from build123d import *

# Parameters (mm, degrees)
SKETCH1_W           = 164.845307866
SKETCH1_H           = 115.711925012
SKETCH1_W_2         = 150.387290324
SKETCH1_H_2         = 105.563228254
BOSS_EXTRUDE1_DEPTH = 2.54
SKETCH1_3_W         = 164.845307866
SKETCH1_3_H         = 115.711925012
SKETCH1_3_W_2       = 150.387290324
SKETCH1_3_H_2       = 105.563228254
BOSS_EXTRUDE2_DEPTH = 53.34
BOSS_EXTRUDE3_START = 53.34
SKETCH1_4_W         = 164.845307866
SKETCH1_4_H         = 115.711925012
SKETCH1_4_W_2       = 150.387290324
SKETCH1_4_H_2       = 105.563228254
BOSS_EXTRUDE3_DEPTH = 2.54
SKETCH2_R           = 31.968042231
SKETCH2_R_2         = 7.197604608
SKETCH2_R_3         = 7.702224934
SKETCH2_W           = 12.372659968
SKETCH2_H           = 29.724433098
CUT_EXTRUDE1_DEPTH  = 2.54
SKETCH3_W           = 4.472305678
SKETCH3_H           = 33.780947159
SKETCH3_W_2         = 4.478852124
SKETCH3_W_3         = 5.014326271
SKETCH3_W_4         = 5.285336568
SKETCH3_W_5         = 5.288609791
SKETCH3_W_6         = 4.762955313
SKETCH3_W_7         = 4.703323858
SKETCH3_W_8         = 4.457199363
CUT_EXTRUDE2_DEPTH  = 81.820687539


with BuildPart() as part:
    # Sketch1 → Boss-Extrude1 (new body)
    with BuildSketch(Plane(origin=(0, 0, 0), x_dir=(1, 0, 0), z_dir=(0, 1, 0))):
        Rectangle(SKETCH1_W, SKETCH1_H)
        Rectangle(SKETCH1_W_2, SKETCH1_H_2, mode=Mode.SUBTRACT)
        Rectangle(SKETCH1_W_2, SKETCH1_H_2)
    extrude(amount=BOSS_EXTRUDE1_DEPTH)

    # Sketch1<3> → Boss-Extrude2 (add)
    with BuildSketch(Plane(origin=(0, 0, 0), x_dir=(1, 0, 0), z_dir=(0, 1, 0))):
        Rectangle(SKETCH1_3_W, SKETCH1_3_H)
        Rectangle(SKETCH1_3_W_2, SKETCH1_3_H_2, mode=Mode.SUBTRACT)
    extrude(amount=BOSS_EXTRUDE2_DEPTH)

    # Sketch1<4> → Boss-Extrude3 (add)
    with BuildSketch(Plane(origin=(0, 0, 0), x_dir=(1, 0, 0), z_dir=(0, 1, 0)).offset(BOSS_EXTRUDE3_START)):
        Rectangle(SKETCH1_4_W, SKETCH1_4_H)
        Rectangle(SKETCH1_4_W_2, SKETCH1_4_H_2, mode=Mode.SUBTRACT)
        Rectangle(SKETCH1_4_W_2, SKETCH1_4_H_2)
    extrude(amount=BOSS_EXTRUDE3_DEPTH)

    # Sketch2 → Cut-Extrude1 (cut)
    with BuildSketch(Plane(origin=(0, 55.88, 0), x_dir=(1, 0, 0), z_dir=(0, 1, 0))):
        with Locations(Location((27.35736774, 0, 0), (0, 0, 270))):
            Circle(SKETCH2_R)
        with Locations(Location((-29.22455859, 32.289622442, 0), (0, 0, 270))):
            Circle(SKETCH2_R_2)
        with Locations(Location((-29.22455859, 3.70269924, 0), (0, 0, 270))):
            Circle(SKETCH2_R_2)
        with Locations(Location((-55.407149161, -25.489564673, 0), (0, 0, 270))):
            Circle(SKETCH2_R_3)
        with Locations((-55.407149161, 14.862216549)):
            Rectangle(SKETCH2_W, SKETCH2_H)
    extrude(amount=-CUT_EXTRUDE1_DEPTH, mode=Mode.SUBTRACT)

    # Sketch3 → Cut-Extrude2 (cut, along a direction that is not the sketch's normal)
    with BuildSketch(Plane.XY.offset(57.855962506)):
        with Locations((65.530463392, 25.643218911)):
            Rectangle(SKETCH3_W, SKETCH3_H)
        with Locations((56.86140712, 25.643218911)):
            Rectangle(SKETCH3_W_2, SKETCH3_H)
        with Locations((47.101763215, 25.643218911)):
            Rectangle(SKETCH3_W_3, SKETCH3_H)
        with Locations((37.06783579, 25.643218911)):
            Rectangle(SKETCH3_W_2, SKETCH3_H)
        with Locations((26.637212589, 25.643218911)):
            Rectangle(SKETCH3_W_4, SKETCH3_H)
        with Locations((16.066174405, 25.643218911)):
            Rectangle(SKETCH3_W_5, SKETCH3_H)
        with Locations((5.491862999, 25.643218911)):
            Rectangle(SKETCH3_W_6, SKETCH3_H)
        with Locations((-4.645950069, 25.643218911)):
            Rectangle(SKETCH3_W_7, SKETCH3_H)
        with Locations((-14.58703369, 25.643218911)):
            Rectangle(SKETCH3_W_8, SKETCH3_H)
    extrude(amount=-CUT_EXTRUDE2_DEPTH, dir=(0.7071067811865475, 0, 0.7071067811865477), mode=Mode.SUBTRACT)


solid = part.part
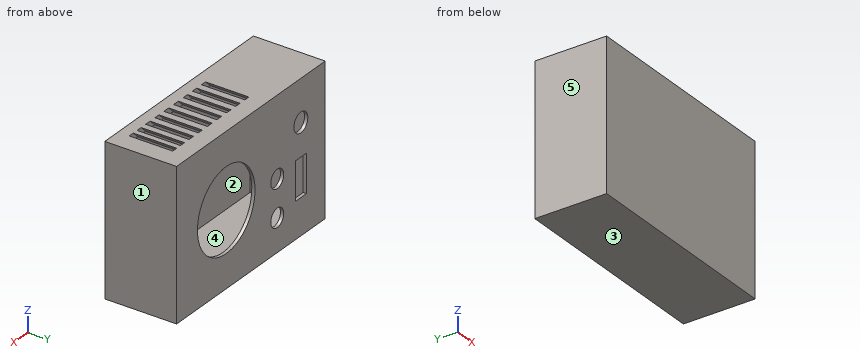
The listing builds one solid part. Answer for the finished solid, in the listing's coordinates (mm). Face numbers are marked on the shaded views. A direction names the side the tool comes from. Coordinates: 2 decimals unless noted, no trailing zeros. Order: outer loops, then holes, each group sorted by start corner. A loop starts at its lowest first (then second) coordinate and runs counter-clockwise, first axis right, second up. Notation, with made-up numbers: (81, 89.25) -> (106, 89.25) arc R35 ccw to (106, 125.25) -> close; hole circle Ø2 at (85.5, 83). An arc over 180 degrees is marked (long way). Answer in a Markdown table with one row per item. Add a question column.
Item 1: Find section C-C (y = 4.5). Write down the section's boundary in (x, z).
Item 2: Find section A-A (x = -20). Write down the section's boundary in (y, z).
Item 3: Which of the six approach directions +Z, -Z, +X, -X, +Y, -Y give full straight-line access (tool end or side, diameter ignored) to the marked faces 1 and 2?
Item 4: Find section B-B (z = -2). Write down the section's boundary in (x, y), then the cut area to 3 significant figures.
Item 5: Find section D-D (y = 31). State how many separate pieces and enclosed holes the cut face has, then the cut area to 3 significant figures.
Item 6: This flat-tipped pin is pushed along its axis until it touches: P1, Ø8.5, axis at x = -29.22, z = -3.7, coming from the +Y side. Where does it stop, or does it pass through?
Item 7: Find the intervals of material crossed by L1, parallel to Y at x = 66, z = -14.5; L2, parallel to Z at x = -33.5, y = 13.5; L3, parallel to X at y = 11.5, z = -26.5, in increasing order. Write a range as from..to.
Item 8: Determine the mould class of the marked faces 3, 4 and 5 for opening direction Z: +Z half, -Z half, draft (parallel to the pull), parting line (faces both ways), or undercut.
Result set:
| question | item | result |
|---|---|---|
| 1 | outline | (-82.42, -57.86) -> (82.42, -57.86) -> (82.42, 57.86) -> (-82.42, 57.86) -> close; hole (-75.19, -52.78) -> (75.19, -52.78) -> (75.19, 52.78) -> (-75.19, 52.78) -> close |
| 2 | outline | (0, -57.86) -> (55.88, -57.86) -> (55.88, 57.86) -> (0, 57.86) -> close; hole (2.54, -52.78) -> (53.34, -52.78) -> (53.34, 52.78) -> (42.53, 52.78) -> (42.53, 54.67) -> (8.75, 54.67) -> (8.75, 52.78) -> (2.54, 52.78) -> close |
| 3 | face 1 | +Z, -Z, +X, +Y, -Y |
| 3 | face 2 | none |
| 4 | outline | (-82.42, 0) -> (82.42, 0) -> (82.42, 55.88) -> (59.26, 55.88) -> (59.26, 53.34) -> (75.19, 53.34) -> (75.19, 2.54) -> (-75.19, 2.54) -> (-75.19, 53.34) -> (-61.59, 53.34) -> (-61.59, 55.88) -> (-82.42, 55.88) -> close; (-49.22, 53.34) -> (-36.22, 53.34) -> (-36.22, 55.88) -> (-49.22, 55.88) -> close; (-22.23, 53.34) -> (-4.55, 53.34) -> (-4.55, 55.88) -> (-22.23, 55.88) -> close |
| 4 | area | 1,340 mm² |
| 5 | separate pieces | 9 |
| 5 | enclosed holes | 0 |
| 5 | area | 2,980 mm² |
| 6 | P1 | stops at y = 2.54 |
| 7 | L1 | y = 0..2.54, 53.34..55.88 |
| 7 | L2 | z = -57.86..-52.78, 52.78..57.86 |
| 7 | L3 | x = -82.42..-75.19, 75.19..82.42 |
| 8 | face 3 | -Z half |
| 8 | face 4 | undercut |
| 8 | face 5 | draft |
